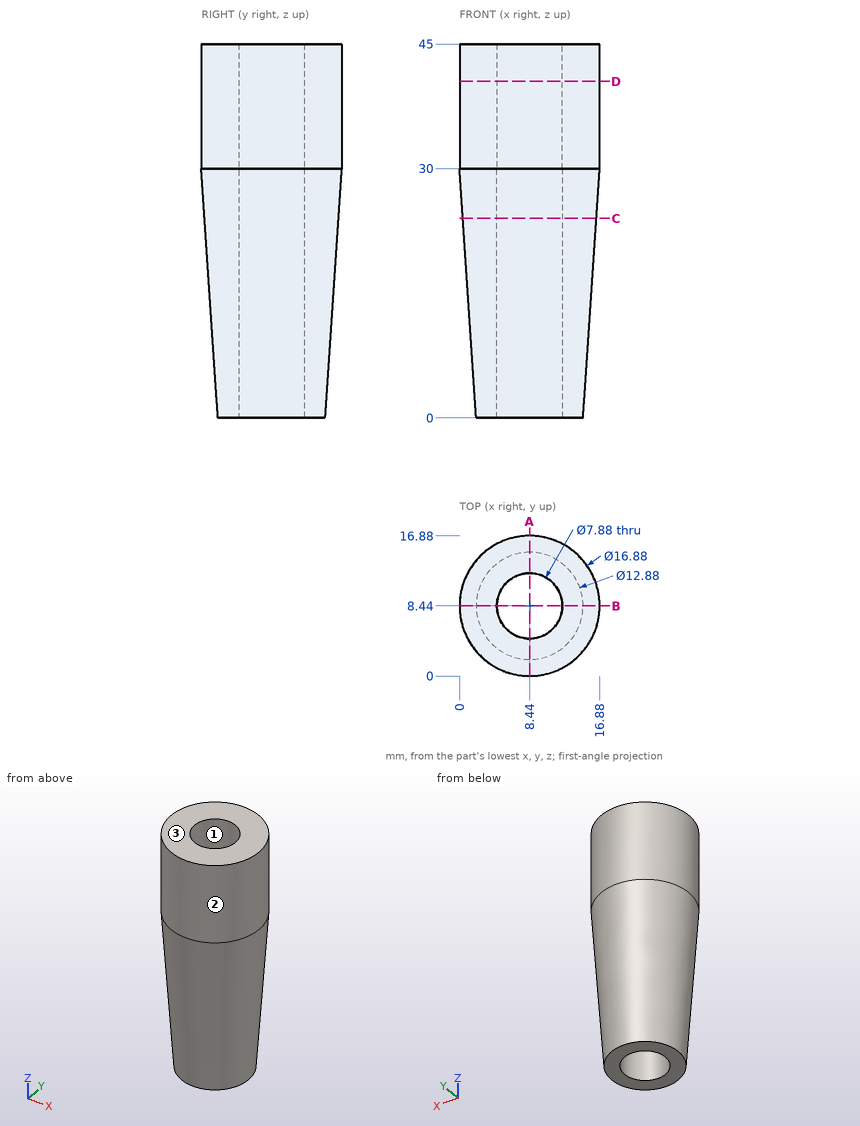
Can you work these out from the drawing? Everything is in mm from the part's minimum corner. Coordinates: 2 decimals unless noted, no trailing zeros. Loops run counter-clockwise (first coordinate to the right, second up) from the corner with the lowest first, then second, coordinate; pieces in that order, holes last.
1) Please list where these lines run through material, in increasing order: line 1 along Y through (x, z) = (8.44, 34.5); line 2 along Y through (x, z) = (7.5, 42).
Reported:
line 1: y = 0 to 4.5, 12.38 to 16.88
line 2: y = 0.05 to 4.61, 12.27 to 16.83
2) Will these pins go through, and if not, where does the flat tip stop? pin 1 Ø4 at (y, z) = (13, 38) entering from -X; pin 2 Ø2 at (x, z) = (15, 27.5) entering from +Y; pin 3 Ø10 at (x, z) = (9, 29.5) entering from +Y; pin 4 Ø6 at (y, z) = (11.5, 12.5) entering from +X.
Reported:
pin 1: stops at x = 0.4
pin 2: stops at y = 14.57
pin 3: stops at y = 16.88
pin 4: stops at x = 15.8
3) Imagine slicing it at A-A (x = 8.44). List the corners of the cut face in (y, z) for me, and give its area (3 significant figures).
Reported:
outline: (0, 30) - (2, 0) - (4.5, 0) - (4.5, 45) - (0, 45) - close; (12.38, 0) - (14.88, 0) - (16.88, 30) - (16.88, 45) - (12.38, 45) - close
area: 345 mm2
4) Imagine slicing it at D-D (z = 40.5). List the corners of the cut face in (x, y) for me.
Reported:
outline: circle Ø16.88 at (8.44, 8.44); hole circle Ø7.88 at (8.44, 8.44)
5) Imagine slicing it at C-C (z = 24). List the corners of the cut face in (x, y) for me.
Reported:
outline: circle Ø16.08 at (8.44, 8.44); hole circle Ø7.88 at (8.44, 8.44)
6) Thinking about a two-plate mould opening in Y: for the marked faces 1, 2 and 3, which applies, released by +Y, released by -Y, zero draft, split by the parting line, or undercut?
Reported:
face 1: undercut
face 2: split by the parting line
face 3: zero draft
